Model file for the job. Use its own axes, mm. A direction names the side the tool comes from. Coordinates: 2 decimals unless noted, no trailing zeros. Order: outer loops, then holes, each group sorted by start corner. A loop starts at its lowest first (then second) coordinate and runs counter-clockwise, first axis right, second up.
from build123d import *

# Parameters (mm, degrees)
EXTRUDE_1_DEPTH = 10
EXTRUDE_2_DEPTH = 20
SKETCH_1_4_R    = 32.5
SKETCH_1_4_R_2  = 5
SKETCH_1_4_R_3  = 9
SKETCH_1_4_R_4  = 47
SKETCH_1_4_R_5  = 6
EXTRUDE_3_DEPTH = 30
SKETCH_1_5_R    = 19
EXTRUDE_4_DEPTH = 20


with BuildPart() as part:
    # Sketch 1 → Extrude 1 (new body)
    with BuildSketch(Plane.XY):
        with BuildLine():
            ThreePointArc((-45.198702821, 12.887096774), (-28.313481344, 37.514620806), (0, 47))
            Line((0, 47), (-205, 47))
            ThreePointArc((-205, 47), (-200.606601718, 36.393398282), (-190, 32))
            Line((-190, 32), (-178, 32))
            ThreePointArc((-178, 32), (-174.464466094, 30.535533906), (-173, 27))
            Line((-173, 27), (-173, -58))
            ThreePointArc((-173, -58), (-168.606601718, -68.606601718), (-158, -73))
            Line((-158, -73), (-126.369910086, -73))
            ThreePointArc((-126.369910086, -73), (-119.574013491, -74.627797882), (-114.253096375, -79.157894737))
            ThreePointArc((-114.253096375, -79.157894737), (-120.019995674, -65.565058581), (-119.177594319, -50.823529412))
            ThreePointArc((-119.177594319, -50.823529412), (-122.780512208, -56.007349565), (-128.770700264, -58))
            Line((-128.770700264, -58), (-143, -58))
            ThreePointArc((-143, -58), (-153.606601718, -53.606601718), (-158, -43))
            Line((-158, -43), (-158, 27))
            ThreePointArc((-158, 27), (-156.535533906, 30.535533906), (-153, 32))
            Line((-153, 32), (-59.623820743, 32))
            ThreePointArc((-59.623820743, 32), (-47.651069422, 26.03621745), (-45.198702821, 12.887096774))
        make_face()
    extrude(amount=EXTRUDE_1_DEPTH)

    # Sketch 1_3 → Extrude 2 (add)
    with BuildSketch(Plane.XY):
        with BuildLine():
            ThreePointArc((-16.3012652, -44.08252208), (-41.915938314, -21.261564271), (-45.198702821, 12.887096774))
            ThreePointArc((-45.198702821, 12.887096774), (-47.651069422, 26.03621745), (-59.623820743, 32))
            Line((-59.623820743, 32), (-153, 32))
            ThreePointArc((-153, 32), (-156.535533906, 30.535533906), (-158, 27))
            Line((-158, 27), (-158, -43))
            ThreePointArc((-158, -43), (-153.606601718, -53.606601718), (-143, -58))
            Line((-143, -58), (-128.770700264, -58))
            ThreePointArc((-128.770700264, -58), (-122.780512208, -56.007349565), (-119.177594319, -50.823529412))
            ThreePointArc((-119.177594319, -50.823529412), (-83.364367108, -27.832300242), (-55.5, -60))
            ThreePointArc((-55.5, -60), (-55.657202848, -63.192721783), (-56.127290608, -66.354557108))
            ThreePointArc((-56.127290608, -66.354557108), (-41.349141883, -46.036566638), (-16.3012652, -44.08252208))
        make_face()
        with BuildLine():
            ThreePointArc((-88.862233392, 15), (-79.271690766, 7.832223886), (-83.429720611, -3.395701572))
            Line((-83.429720611, -3.395701572), (-124.567487218, -30.014256435))
            ThreePointArc((-124.567487218, -30.014256435), (-134.77885301, -30.402777306), (-140, -21.618554864))
            Line((-140, -21.618554864), (-140, 0))
            ThreePointArc((-140, 0), (-135.606601718, 10.606601718), (-125, 15))
            Line((-125, 15), (-88.862233392, 15))
        make_face(mode=Mode.SUBTRACT)
    extrude(amount=EXTRUDE_2_DEPTH)

    # Sketch 1_4 → Extrude 3 (add)
    # profile 1 of 2: a face of its own
    with BuildSketch(Plane.XY):
        with Locations(Location((-88, -60, 0), (0, 0, 163.599314088))):
            Circle(SKETCH_1_4_R)
        with Locations((-78, -42.679491924)):
            Circle(SKETCH_1_4_R_2, mode=Mode.SUBTRACT)
        with Locations((-98, -42.679491924)):
            Circle(SKETCH_1_4_R_2, mode=Mode.SUBTRACT)
        with Locations((-108, -60)):
            Circle(SKETCH_1_4_R_2, mode=Mode.SUBTRACT)
        with Locations((-98, -77.320508076)):
            Circle(SKETCH_1_4_R_2, mode=Mode.SUBTRACT)
        with Locations((-78, -77.320508076)):
            Circle(SKETCH_1_4_R_2, mode=Mode.SUBTRACT)
        with Locations((-68, -60)):
            Circle(SKETCH_1_4_R_2, mode=Mode.SUBTRACT)
        with Locations((-88, -60)):
            Circle(SKETCH_1_4_R_3, mode=Mode.SUBTRACT)
    # profile 2 of 2: a face of its own
    with BuildSketch(Plane.XY):
        with Locations(Location((0, 0, 0), (0, 0, 164.086039314))):
            Circle(SKETCH_1_4_R_4)
        with Locations((-26.162950904, 26.162950904)):
            Circle(SKETCH_1_4_R_5, mode=Mode.SUBTRACT)
        with Locations((-37, 0)):
            Circle(SKETCH_1_4_R_5, mode=Mode.SUBTRACT)
        with Locations((-26.162950904, -26.162950904)):
            Circle(SKETCH_1_4_R_5, mode=Mode.SUBTRACT)
        with Locations((0, -37)):
            Circle(SKETCH_1_4_R_5, mode=Mode.SUBTRACT)
        with Locations((26.162950904, -26.162950904)):
            Circle(SKETCH_1_4_R_5, mode=Mode.SUBTRACT)
        with Locations((37, 0)):
            Circle(SKETCH_1_4_R_5, mode=Mode.SUBTRACT)
        with Locations((26.162950904, 26.162950904)):
            Circle(SKETCH_1_4_R_5, mode=Mode.SUBTRACT)
        with Locations((0, 37)):
            Circle(SKETCH_1_4_R_5, mode=Mode.SUBTRACT)
        with BuildLine():
            ThreePointArc((-9.908271773, 35.648648649), (-14.159286998, 34.183542703), (-18.201195039, 32.21360736))
            ThreePointArc((-18.201195039, 32.21360736), (-19.091883092, 19.091883092), (-32.21360736, 18.201195039))
            ThreePointArc((-32.21360736, 18.201195039), (-34.183542703, 14.159286998), (-35.648648649, 9.908271773))
            ThreePointArc((-35.648648649, 9.908271773), (-27, 0), (-35.648648649, -9.908271773))
            ThreePointArc((-35.648648649, -9.908271773), (-34.183542703, -14.159286998), (-32.21360736, -18.201195039))
            ThreePointArc((-32.21360736, -18.201195039), (-19.091883092, -19.091883092), (-18.201195039, -32.21360736))
            ThreePointArc((-18.201195039, -32.21360736), (-14.159286998, -34.183542703), (-9.908271773, -35.648648649))
            ThreePointArc((-9.908271773, -35.648648649), (0, -27), (9.908271773, -35.648648649))
            ThreePointArc((9.908271773, -35.648648649), (14.159286998, -34.183542703), (18.201195039, -32.21360736))
            ThreePointArc((18.201195039, -32.21360736), (19.091883092, -19.091883092), (32.21360736, -18.201195039))
            ThreePointArc((32.21360736, -18.201195039), (34.183542703, -14.159286998), (35.648648649, -9.908271773))
            ThreePointArc((35.648648649, -9.908271773), (27, 0), (35.648648649, 9.908271773))
            ThreePointArc((35.648648649, 9.908271773), (34.183542703, 14.159286998), (32.21360736, 18.201195039))
            ThreePointArc((32.21360736, 18.201195039), (19.091883092, 19.091883092), (18.201195039, 32.21360736))
            ThreePointArc((18.201195039, 32.21360736), (14.159286998, 34.183542703), (9.908271773, 35.648648649))
            ThreePointArc((9.908271773, 35.648648649), (0, 27), (-9.908271773, 35.648648649))
        make_face(mode=Mode.SUBTRACT)
    extrude(amount=EXTRUDE_3_DEPTH)

    # Sketch 1_5 → Extrude 4 (add)
    with BuildSketch(Plane.XY):
        with BuildLine():
            ThreePointArc((9.908271773, 35.648648649), (0, 27), (-9.908271773, 35.648648649))
            ThreePointArc((-9.908271773, 35.648648649), (-14.159286998, 34.183542703), (-18.201195039, 32.21360736))
            ThreePointArc((-18.201195039, 32.21360736), (-19.091883092, 19.091883092), (-32.21360736, 18.201195039))
            ThreePointArc((-32.21360736, 18.201195039), (-34.183542703, 14.159286998), (-35.648648649, 9.908271773))
            ThreePointArc((-35.648648649, 9.908271773), (-27, 0), (-35.648648649, -9.908271773))
            ThreePointArc((-35.648648649, -9.908271773), (-34.183542703, -14.159286998), (-32.21360736, -18.201195039))
            ThreePointArc((-32.21360736, -18.201195039), (-19.091883092, -19.091883092), (-18.201195039, -32.21360736))
            ThreePointArc((-18.201195039, -32.21360736), (-14.159286998, -34.183542703), (-9.908271773, -35.648648649))
            ThreePointArc((-9.908271773, -35.648648649), (0, -27), (9.908271773, -35.648648649))
            ThreePointArc((9.908271773, -35.648648649), (14.159286998, -34.183542703), (18.201195039, -32.21360736))
            ThreePointArc((18.201195039, -32.21360736), (19.091883092, -19.091883092), (32.21360736, -18.201195039))
            ThreePointArc((32.21360736, -18.201195039), (34.183542703, -14.159286998), (35.648648649, -9.908271773))
            ThreePointArc((35.648648649, -9.908271773), (27, 0), (35.648648649, 9.908271773))
            ThreePointArc((35.648648649, 9.908271773), (34.183542703, 14.159286998), (32.21360736, 18.201195039))
            ThreePointArc((32.21360736, 18.201195039), (19.091883092, 19.091883092), (18.201195039, 32.21360736))
            ThreePointArc((18.201195039, 32.21360736), (14.159286998, 34.183542703), (9.908271773, 35.648648649))
        make_face()
        Circle(SKETCH_1_5_R, mode=Mode.SUBTRACT)
    extrude(amount=EXTRUDE_4_DEPTH)


solid = part.part
Q1. Mould opens along Y. For faces 4 (the face through (-81, -6, 0)), 5 (the face through (-142, -73, 5)), 6 (the face through (-135.72, 10.49, 9.86)) say: pulls with the +Y half, pulls with the -Y half, needs draft (parallel to the pull), parting line crosses it, or undercut.
Established:
face 4: needs draft
face 5: pulls with the -Y half
face 6: undercut
Q2. Drop flat-ended pins along their axis: P1, Ø2, axis at x = -24.5, z = 22.5, coming from the -Y side; P2, Ø4, axis at x = -20, z = 7, coming from the -Y side; P3, Ø6, axis at x = -108.5, z = 7, coming from the -Y side. Give the stop position or say it passes through.
Established:
P1: stops at y = -40.7
P2: stops at y = -43.51
P3: stops at y = -87.39
Q3. Probe line 1 (Y direction, x = 0, z = 11.75); line 2 (X direction, y = 25, z = 18.5); line 3 (Y direction, x = 4, z = 17.5). List the from-to ranges inside material, lowest first.
Established:
line 1: y = -47 to -43, -31 to -19, 19 to 31, 43 to 47
line 2: x = -158 to -46.94, -39.8 to -32.05, -20.28 to 20.28, 32.05 to 39.8
line 3: y = -46.83 to -41.47, -32.53 to -18.57, 18.57 to 32.53, 41.47 to 46.83
Q4. Cut at B-B, the plane z = 14.25. Count the separate pieces of the cut face and the enclosed holes in it, plus the area to 3 significant figures.
Established:
separate pieces: 1
enclosed holes: 17
area: 14,200 mm2
Q5. Cut at C-C, the plane x = -108. List the corners of the cut face in (y, z), plus the area to 3 significant figures.
Established:
outline: (-85.62, 0) - (-65, 0) - (-65, 30) - (-85.62, 30) - close; (-55, 0) - (-19.29, 0) - (-19.29, 20) - (-34.38, 20) - (-34.38, 30) - (-55, 30) - close; (15, 0) - (47, 0) - (47, 10) - (32, 10) - (32, 20) - (15, 20) - close
area: 2,030 mm2
Q6. Cut at A-A, the plane x = -68. List the corners of the cut face in (y, z), plus the area to 3 significant figures.
Established:
outline: (-85.62, 0) - (-65, 0) - (-65, 30) - (-85.62, 30) - close; (-55, 0) - (47, 0) - (47, 10) - (32, 10) - (32, 20) - (-34.38, 20) - (-34.38, 30) - (-55, 30) - close
area: 2,710 mm2
Q7. Which spindle directions (+Z, -Z, +X, -X, +Y, -Y) get a long thin tool onto all of the face, cutting with end or side? Do faces 1 (the face through (-140, -11, 10)), 2 (the face through (-136, -58, 15)), 3 (the face through (-173, -15, 5)). Say none if no direction does.
Established:
face 1: +Z, -Z
face 2: +Z, -X, -Y
face 3: +Z, -Z, -X, -Y
